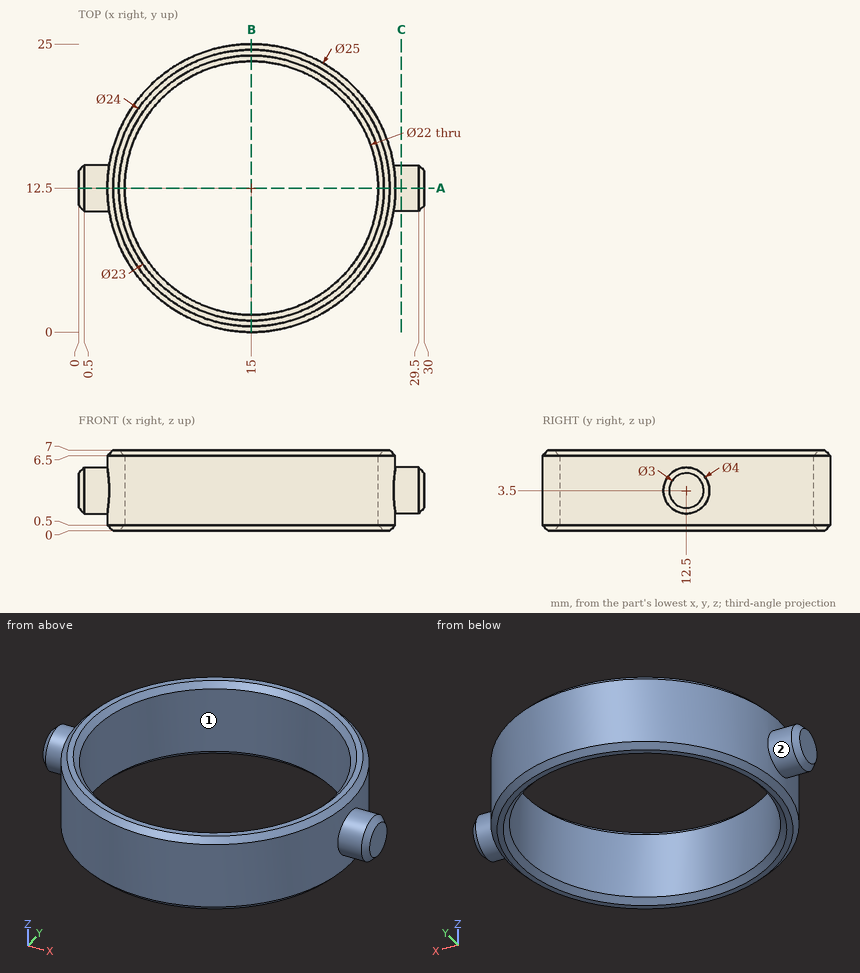
Part print with two shaded views. Sizes in mm from the minimum x, y, z corner. Give positions to 0.01 mm unless a question says otherwise; leave off trailing zeros. Order: outer loops, then holes, each group sorted by start corner. A loop starts at its lowest first (then second) coordinate and runs counter-clockwise, first axis right, second up. Notation, with made-up numbers: M 15,65 L 27,65 A33 ccw 27,93 Z; hole C 29.5,29.25 d8. An arc over 180 degrees is marked long. Use one line per item in the form item = value.
1) Saw through at A-A (y = 12.5). Give the cut face in (x, z), plus the area to 3 significant figures.
Calculated:
outline = M 0,2 L 0.5,1.5 L 2.5,1.5 L 2.5,0.5 L 3,0 L 3.5,0 L 4,0.5 L 4,6.5 L 3.5,7 L 3,7 L 2.5,6.5 L 2.5,5.5 L 0.5,5.5 L 0,5 Z; M 26,0.5 L 26.5,0 L 27,0 L 27.5,0.5 L 27.5,1.5 L 29.5,1.5 L 30,2 L 30,5 L 29.5,5.5 L 27.5,5.5 L 27.5,6.5 L 27,7 L 26.5,7 L 26,6.5 Z
area = 39.5 mm2
2) Two-plate mould, pull along Y, no slides. Class the marked faces 1 and 2: released by +Y, released by -Y, zero draft, split by the parting line, or undercut.
Calculated:
face_1 = undercut
face_2 = split by the parting line
3) Saw through at B-B (x = 15). Give the cut face in (y, z), plus the area to 3 significant figures.
Calculated:
outline = M 0,0.5 L 0.5,0 L 1,0 L 1.5,0.5 L 1.5,6.5 L 1,7 L 0.5,7 L 0,6.5 Z; M 23.5,0.5 L 24,0 L 24.5,0 L 25,0.5 L 25,6.5 L 24.5,7 L 24,7 L 23.5,6.5 Z
area = 20.0 mm2
4) Saw through at C-C (x = 28). Give the cut face in (y, z).
Calculated:
outline = C 12.5,3.5 d4
5) Probe probe 1 along Y at (x, z) = (15, 5.1); probe 2 along Y at (x, z) = (13.25, 1); probe 3 along X at (y, z) = (21, 4.75). List the from-to ranges inside material, lowest first.
Calculated:
probe_1 = 0 to 1.5, 23.5 to 25
probe_2 = 0.12 to 1.64, 23.36 to 24.88
probe_3 = 5.83 to 8.02, 21.98 to 24.17
6) Drop flat-ended pins along their axis: pin 1 (2 mm diameter, centred on y = 3.5, z = 3.5, fed in from -X); pin 2 (1 mm diameter, centred on x = 23.5, z = 3, fed in from -Y); pin 3 (2 mm diameter, centred on x = 3, z = 1.5, fed in from -Y). Give the stop position or say it passes through.
Calculated:
pin_1 = 5.4
pin_2 = 2.9
pin_3 = 6.56
